Model file for the job. Use its own axes, mm. Face numbers are marked on the shaded views. A direction names the side the tool comes from. Coordinates: 2 decimals unless noted, no trailing zeros. Write each loop counter-clockwise with the first axis right and the second up, starting at its lowest first coordinate (ties: lowest second). Pieces come first, ordered by that corner, then holes. Notation, with made-up numbers: M 75.5,78 L 128.5,78 A26 cw 128.5,101 Z; hole C 16,-30 d7. An arc over 180 degrees is marked long. One line per question, with ' | ' between items. Start each with the question number.
(1) Tool access for the marked faces 4 and 5: list every direction of +Z, -Z, +X, -X, +Y, -Y with a clear straight run to the whole face (end or side of a thin tool).
(2) Cut at B-B (z = 16). Write the cut outline in (x, y).
(3) Two-plate mould, pull along X, no slides. Class the marked faces 1, 2 and 3: +X half, -X half, draft (parallel to the pull), parting line (faces both ways), or undercut.
(4) Cut at A-A (x = 16). Write the cut outline in (y, z).
(5) Cut at D-D (z = 1.5). Count the separate pieces of the cut face and the enclosed holes in it, plus the area to 3 significant figures.
(6) Flat gauge pins, fed straight in: pin 1 Ø8 at (x, z) = (-12, -15) entering from +Y; pin 2 Ø3 at (x, z) = (14.5, 16.5) entering from -Y. Where does each tip first touch, or does it go through?
(7) Wall check: probe 1 along Z at (x, y) = (-2.5, 2.25); probe 2 along X at (y, z) = (1.35, -16). Give the ranges that are in metal, low to high.
(8) Cut at C-C (y = 3). Write the cut outline in (x, z).
from build123d import *

# Parameters (mm, degrees)
SKETCH1_W           = 42.2
SKETCH1_H           = 42.2
SKETCH1_R           = 1.7
BOSS_EXTRUDE1_DEPTH = 2
SKETCH1_4_W         = 42.2
SKETCH1_4_H         = 42.2
SKETCH1_4_W_2       = 40.2
SKETCH1_4_H_2       = 40.2
BOSS_EXTRUDE2_DEPTH = 10
CUT_EXTRUDE1_DEPTH  = 2
CIRPATTERN1_COUNT   = 4


with BuildPart() as part:
    # Sketch1 → Boss-Extrude1 (new body)
    with BuildSketch(Plane(origin=(0, 0, 0), x_dir=(1, 0, 0), z_dir=(0, 1, 0))):
        Rectangle(SKETCH1_W, SKETCH1_H)
        with Locations(Location((16, 16, 0), (0, 0, 270))):
            Circle(SKETCH1_R, mode=Mode.SUBTRACT)
        with Locations(Location((16, -16, 0), (0, 0, 270))):
            Circle(SKETCH1_R, mode=Mode.SUBTRACT)
        with Locations(Location((-16, -16, 0), (0, 0, 270))):
            Circle(SKETCH1_R, mode=Mode.SUBTRACT)
        with Locations(Location((-16, 16, 0), (0, 0, 270))):
            Circle(SKETCH1_R, mode=Mode.SUBTRACT)
    extrude(amount=BOSS_EXTRUDE1_DEPTH)

    # Sketch1<4> → Boss-Extrude2 (add)
    with BuildSketch(Plane(origin=(0, 0, 0), x_dir=(1, 0, 0), z_dir=(0, 1, 0))):
        Rectangle(SKETCH1_4_W, SKETCH1_4_H)
        Rectangle(SKETCH1_4_W_2, SKETCH1_4_H_2, mode=Mode.SUBTRACT)
    extrude(amount=BOSS_EXTRUDE2_DEPTH)

    # Sketch1<5> → Cut-Extrude1 (cut)
    with BuildSketch(Plane(origin=(0, 0, 0), x_dir=(1, 0, 0), z_dir=(0, 1, 0))):
        with BuildLine():
            ThreePointArc((12.823589374, 0.5), (9.074537025, 9.074537025), (0.5, 12.823589374))
            Line((0.5, 12.823589374), (0.5, 7.14920353))
            ThreePointArc((0.5, 7.14920353), (5.067598599, 5.067598599), (7.14920353, 0.5))
            Line((7.14920353, 0.5), (12.823589374, 0.5))
        make_face()
        with BuildLine():
            ThreePointArc((6.146362972, 0.5), (4.360491817, 4.360491817), (0.5, 6.146362972))
            Line((0.5, 6.146362972), (0.5, 0.5))
            Line((0.5, 0.5), (6.146362972, 0.5))
        make_face()
        with BuildLine():
            Line((0.5, 19.993749023), (0.5, 13.824294236))
            ThreePointArc((0.5, 13.824294236), (9.781643806, 9.781643806), (13.824294236, 0.5))
            Line((13.824294236, 0.5), (19.993749023, 0.5))
            ThreePointArc((19.993749023, 0.5), (14.142135624, 14.142135624), (0.5, 19.993749023))
        make_face()
    cut_extrude1 = extrude(amount=CUT_EXTRUDE1_DEPTH, mode=Mode.SUBTRACT)

    # CirPattern1: Cut-Extrude1 ×4 about axis
    cirpattern1_axis = Axis((0, 0, 0), (0, 1, 0))
    for i in range(1, CIRPATTERN1_COUNT):
        add(cut_extrude1.rotate(cirpattern1_axis, i * 360 / CIRPATTERN1_COUNT), mode=Mode.SUBTRACT)


solid = part.part
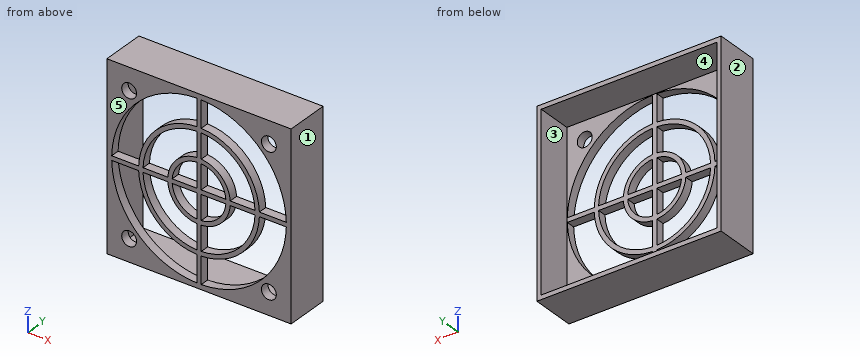
Filled in:
1) face 4: +Y | face 5: +Z, -Z, +X, -X, -Y
2) outline: M -21.1,0 L -17.7,0 L -17.7,2 L -20.1,2 L -20.1,10 L -21.1,10 Z; M -14.3,0 L -12,0 L -12,2 L -14.3,2 Z; M -0.5,0 L 0.5,0 L 0.5,2 L -0.5,2 Z; M 12,0 L 14.3,0 L 14.3,2 L 12,2 Z; M 17.7,0 L 21.1,0 L 21.1,10 L 20.1,10 L 20.1,2 L 17.7,2 Z
3) face 1: +X half | face 2: -X half | face 3: undercut
4) outline: M 0,-21.1 L 10,-21.1 L 10,-20.1 L 2,-20.1 L 2,-17.7 L 0,-17.7 Z; M 0,-14.3 L 2,-14.3 L 2,-12 L 0,-12 Z; M 0,-0.5 L 2,-0.5 L 2,0.5 L 0,0.5 Z; M 0,12 L 2,12 L 2,14.3 L 0,14.3 Z; M 0,17.7 L 2,17.7 L 2,20.1 L 10,20.1 L 10,21.1 L 0,21.1 Z
5) separate pieces: 7 | enclosed holes: 0 | area: 30.8 mm²
6) pin 1: y = 2 | pin 2: y = 0
7) probe 1: -21.1 to -20.1, 20.1 to 21.1 | probe 2: -21.1 to -17.7, -14.3 to -12, -0.5 to 0.5, 12 to 14.3, 17.7 to 21.1
8) outline: M -21.1,-21.1 L 21.1,-21.1 L 21.1,21.1 L -21.1,21.1 Z; hole M -20.1,-20.1 L 20.1,-20.1 L 20.1,20.1 L -20.1,20.1 Z
